Verification items for the finished model (mm, model axes). A direction names the side the tool comes from. Round coordinates to 2 decimals unless told otherwise and drop trailing zeros. Order: outer loops, then holes, each group sorted by start corner. A loop starts at its lowest first (then second) coordinate and runs counter-clockwise, first axis right, second up. Notation, with made-up numbers: (1.5, -18.75) -> (15.5, -18.75) arc R17 ccw to (15.5, 1.25) -> close; hole circle Ø4 at (-37.75, 10.25). An arc over 180 degrees is marked (long way). Put each result on its own line as item: value.
```python
from build123d import *

# Parameters (mm, degrees)
SKETCH1_W               = 3.175
SKETCH1_H               = 69.74205
CUT_EXTRUDE1_DEPTH      = 25.146
CUT_EXTRUDE1_DEPTH_BACK = 108.204
SKETCH2_R               = 6.35


with BuildPart() as part:
    # Sketch1 → Revolve1 (revolve)
    with BuildSketch(Plane.XY, mode=Mode.PRIVATE) as revolve1_sk:
        Polygon((13.238453462, 31.037681507), (0, 76.09205), (0, 6.35), (22.013333333, 6.35), (40.64, 6.35), (40.64, 76.09205), (27.401546538, 31.037681507), align=None)
        with Locations((-1.5875, 41.221025)):
            Rectangle(SKETCH1_W, SKETCH1_H)
        with Locations((42.2275, 41.221025)):
            Rectangle(SKETCH1_W, SKETCH1_H)
    revolve(revolve1_sk.sketch.rotate(Axis((0, 0, 0), (1, 0, 0)), 90), axis=Axis((0, 0, 0), (1, 0, 0)))

    # Sketch2 → Cut-Extrude1 (cut, two sides: drawn at the far end of the back side and taken through both)
    # profile 1 of 4: a face of its own
    with BuildSketch(Plane(origin=(43.815, 0, 0), x_dir=(0, 0, -1), z_dir=(1, 0, 0)).offset(-CUT_EXTRUDE1_DEPTH_BACK)):
        with BuildLine():
            Line((3.175, 12.296722124), (3.175, 9.525))
            Line((3.175, 9.525), (-3.175, 9.525))
            Line((-3.175, 9.525), (-3.175, 12.296722124))
            ThreePointArc((-3.175, 12.296722124), (-7.777129933, -10.040231571), (12.7, 0))
            ThreePointArc((12.7, 0), (10.040231571, 7.777129933), (3.175, 12.296722124))
        make_face()
        Circle(SKETCH2_R, mode=Mode.SUBTRACT)
    # profile 2 of 4: a face of its own
    with BuildSketch(Plane(origin=(43.815, 0, 0), x_dir=(0, 0, -1), z_dir=(1, 0, 0)).offset(-CUT_EXTRUDE1_DEPTH_BACK)):
        with BuildLine():
            Line((-3.175, 9.525), (3.175, 9.525))
            Line((3.175, 9.525), (3.175, 12.296722124))
            ThreePointArc((3.175, 12.296722124), (0, 12.7), (-3.175, 12.296722124))
            Line((-3.175, 12.296722124), (-3.175, 9.525))
        make_face()
    # profile 3 of 4: a face of its own
    with BuildSketch(Plane(origin=(43.815, 0, 0), x_dir=(0, 0, -1), z_dir=(1, 0, 0)).offset(-CUT_EXTRUDE1_DEPTH_BACK)):
        with BuildLine():
            ThreePointArc((-3.175, 12.296722124), (0, 12.7), (3.175, 12.296722124))
            Line((3.175, 12.296722124), (3.175, 15.875))
            Line((3.175, 15.875), (-3.175, 15.875))
            Line((-3.175, 15.875), (-3.175, 12.296722124))
        make_face()
    # profile 4 of 4: a face of its own
    with BuildSketch(Plane(origin=(43.815, 0, 0), x_dir=(0, 0, -1), z_dir=(1, 0, 0)).offset(-CUT_EXTRUDE1_DEPTH_BACK)):
        with BuildLine():
            Line((-3.175, 9.525), (3.175, 9.525))
            Line((3.175, 9.525), (3.175, 12.296722124))
            ThreePointArc((3.175, 12.296722124), (0, 12.7), (-3.175, 12.296722124))
            Line((-3.175, 12.296722124), (-3.175, 9.525))
        make_face()
    extrude(amount=CUT_EXTRUDE1_DEPTH + CUT_EXTRUDE1_DEPTH_BACK, mode=Mode.SUBTRACT)


solid = part.part
```
Item 1: Sectioned sample at C-C, the plane x = 9. Record the boundary of the cut face in (y, z) (3 decimals), then the cut area to 3 significant figures.
Geometry check:
outline: circle Ø90.925 at (0, 0); hole (12.297, -3.175) -> (15.875, -3.175) -> (15.875, 3.175) -> (12.297, 3.175) arc R12.7 ccw (long way) to start
area: 5,970 mm2
Item 2: Release check for a two-part mould opening along X. For faces 4 (the face through (12.4, 33.1, -7.3)), 5 (the face through (43.815, -1, -16)), 6 (the face through (42.25, -75.445, -9.906)) record: pulls with the +X half, pulls with the -X half, needs draft (parallel to the pull), parting line crosses it, or undercut.
Geometry check:
face 4: undercut
face 5: pulls with the +X half
face 6: needs draft
Item 3: Tool access check on faces 1 (the face through (28.044, -9.98, 31.691)), 2 (the face through (20, 14, 3.175)), 3 (the face through (-3.175, -1, -16)). Record the directions out of +Z, -Z, +X, -X, +Y, -Y that give a thin tool (end or side, any length) a straight path to the whole face; none if there is none.
Geometry check:
face 1: none
face 2: +X, -X
face 3: +Z, -Z, -X, +Y, -Y
Item 4: Sectioned sample at B-B, the plane x = 22.5. Record the boundary of the cut face in (y, z) (3 decimals).
Geometry check:
outline: circle Ø62.075 at (0, 0); hole (12.297, -3.175) -> (15.875, -3.175) -> (15.875, 3.175) -> (12.297, 3.175) arc R12.7 ccw (long way) to start
Item 5: Sectioned sample at A-A, the plane z = 0. Record the boundary of the cut face in (x, y) (3 decimals), then the cut area to 3 significant figures.
Geometry check:
outline: (-3.175, -76.092) -> (0, -76.092) -> (13.238, -31.038) -> (27.402, -31.038) -> (40.64, -76.092) -> (43.815, -76.092) -> (43.815, -12.7) -> (-3.175, -12.7) -> close; (-3.175, 15.875) -> (43.815, 15.875) -> (43.815, 76.092) -> (40.64, 76.092) -> (27.402, 31.038) -> (13.238, 31.038) -> (0, 76.092) -> (-3.175, 76.092) -> close
area: 3,340 mm2
Item 6: Depth check by flat-ended pin: pin 1 Ø1.8 at (x, y) = (15.5, 15) entering from +Z. Enter the tip coordinate at first touch or a pass-through.
Geometry check:
pin 1: z = 27.65
Item 7: Material ranges on line 1 along Z through (x, y) = (17, -0.5); line 2 along Y through (x, z) = (18, 0) (3 decimals); line 3 along X through (y, z) = (18.5, 47) (3 decimals), recorded low to high.
Geometry check:
line 1: -31.03 to -12.69, 12.69 to 31.03
line 2: -31.038 to -12.7, 15.875 to 31.038
line 3: -3.175 to 7.517, 33.123 to 43.815
